Build history of the part. All positions in model axes, mm. A direction names the side the tool comes from. Give positions to 0.01 mm unless a question says otherwise; leave off trailing zeros. Order: outer loops, then holes, each group sorted by start corner. A loop starts at its lowest first (then second) coordinate and runs counter-clockwise, first axis right, second up. Notation, with made-up numbers: (32, -26) - (84, -26) arc R28 ccw to (84, 8) - close; hole circle Ø3 at (0, -8.75). An arc over 180 degrees is marked (long way). Write each question's results on one line, items separated by ' | '. Start each with the question number.
1) Drop flat-ended pins along their axis: pin 1 Ø10 at (x, y) = (5, 77.5) entering from +Z; pin 2 Ø1 at (x, z) = (21, -539) entering from +Y; pin 3 Ø1 at (x, y) = (33, 150) entering from -Z. Give the stop position or say it passes through.
2) Cut at D-D on z = -394. List the corners of the cut face in (x, y), plus the area to 3 significant figures.
3) Tool access for faces 1 (the face through (19.32, 477.58, -764.5)), 2 (the face through (19, 0, -129)): list every direction of +Z, -Z, +X, -X, +Y, -Y with a clear straight run to the whole face (end or side of a thin tool).
4) Cut at B-B on z = -123.5. List the corners of the cut face in (x, y), plus the area to 3 significant figures.
5) Cut at C-C on y = 472. List the corners of the cut face in (x, z).
6) Drill centre lines: line 1 along Z through (x, y) = (18, 265); line 2 along Y through (x, z) = (20, -766.5); line 3 along Y through (x, z) = (20.5, -819.5). Where is each one in solid material? Low to high. Write a range as from..to.
7) Cut at A-A on x = 29. List the corners of the cut face in (y, z), plus the area to 3 significant figures.
from build123d import *

# Parameters (mm, degrees)
BOSS_EXTRUDE2_DEPTH = 38.1
CUT_EXTRUDE2_REACH  = 573.5
CUT_EXTRUDE3_DEPTH  = 190.5
CUT_EXTRUDE4_DEPTH  = 190.5
CUT_EXTRUDE5_DEPTH  = 190.5


with BuildPart() as part:
    # Sketch1 → Boss-Extrude2 (new body)
    with BuildSketch(Plane(origin=(0, 0, 0), x_dir=(0, 0, -1), z_dir=(1, 0, 0))):
        Polygon((0, 0), (0, 190.5), (372.860234147, 190.5), (372.860234147, 381), (745.720468294, 381), (745.720468294, 571.5), (1109.600446319, 571.5), (1109.600446319, 436.526629402), (255.199284902, 0), align=None)
    extrude(amount=BOSS_EXTRUDE2_DEPTH)

    # Cut-Extrude2: up to this face of the body (flat: up to its plane)
    cut_extrude2_end = Plane(part.part.faces().sort_by_distance((19.05, 218.263314701, -682.399865611))[0])
    # Sketch2 → Cut-Extrude2 (cut, up to the picked face)
    with BuildSketch(Plane(origin=(0, 571.5, 0), x_dir=(1, 0, 0), z_dir=(0, 1, 0)), mode=Mode.PRIVATE) as cut_extrude2_sk1:
        Polygon((38.1, 1109.600446319), (0, 1109.600446319), (38.1, 1071.500446319), align=None)
    cut_extrude2_tool1 = split(extrude(cut_extrude2_sk1.sketch, amount=-CUT_EXTRUDE2_REACH, mode=Mode.PRIVATE), bisect_by=cut_extrude2_end, keep=Keep.BOTH, mode=Mode.PRIVATE)
    add(cut_extrude2_tool1.solids().sort_by_distance((25.4, 571.5, -1096.900446))[0], mode=Mode.SUBTRACT)

    # Sketch2_3 → Cut-Extrude3 (cut)
    with BuildSketch(Plane(origin=(0, 571.5, 0), x_dir=(1, 0, 0), z_dir=(0, 1, 0))):
        Polygon((38.1, 745.720468294), (0, 783.820468294), (0, 745.720468294), align=None)
    extrude(amount=-CUT_EXTRUDE3_DEPTH, mode=Mode.SUBTRACT)

    # Sketch3 → Cut-Extrude4 (cut)
    with BuildSketch(Plane(origin=(0, 381, 0), x_dir=(1, 0, 0), z_dir=(0, 1, 0))):
        Polygon((38.1, 372.860234147), (0, 410.960234147), (0, 372.860234147), align=None)
    extrude(amount=-CUT_EXTRUDE4_DEPTH, mode=Mode.SUBTRACT)

    # Sketch4 → Cut-Extrude5 (cut)
    with BuildSketch(Plane(origin=(0, 190.5, 0), x_dir=(1, 0, 0), z_dir=(0, 1, 0))):
        Polygon((38.1, 0), (0, 38.1), (0, 0), align=None)
    extrude(amount=-CUT_EXTRUDE5_DEPTH, mode=Mode.SUBTRACT)


solid = part.part
Results:
1) pin 1: z = -28.1 | pin 2: y = 381 | pin 3: z = -549.77
2) outline: (0, 70.92) - (38.1, 70.92) - (38.1, 381) - (16.96, 381) - (16.96, 190.5) - (0, 190.5) - close | area: 8,580 mm^2
3) face 1: +Z, -X, +Y | face 2: +Z, -Z, +X, -X, -Y
4) outline: (0, 0) - (38.1, 0) - (38.1, 190.5) - (0, 190.5) - close | area: 7,260 mm^2
5) outline: (0, -1109.6) - (38.1, -1071.5) - (38.1, -745.72) - (0, -783.82) - close
6) line 1: -773.88..-392.96 | line 2: 261.23..571.5 | line 3: 288.31..571.5
7) outline: (0, -255.2) - (421.71, -1080.6) - (571.5, -1080.6) - (571.5, -754.82) - (381, -754.82) - (381, -381.96) - (190.5, -381.96) - (190.5, -9.1) - (0, -9.1) - close | area: 225,000 mm^2
